from build123d import *

# Parameters (mm, degrees)
FILLET1_R = 1.524
FILLET2_R = 0.508


with BuildPart() as part:
    # Sketch3 → Revolve1 (revolve)
    with BuildSketch(Plane(origin=(0, 0, 0), x_dir=(0, 0, -1), z_dir=(1, 0, 0))):
        Polygon((-35.9918, -34.3535), (35.9918, -34.3535), (35.9918, -30.3149), (1.1938, -30.3149), (1.1938, -29.1973), (-1.1938, -29.1973), (-1.1938, -30.3149), (-35.9918, -30.3149), align=None)
    revolve(axis=Axis((0, 0, 35.9918), (0, 0, -1)))

    # Fillet1
    fillet1_edges = [part.edges().sort_by_distance(p)[0] for p in [
        (0, 30.3149, -35.9918),
        (0, 30.3149, 35.9918),
    ]]
    fillet(fillet1_edges, radius=FILLET1_R)

    # Fillet2
    fillet2_edges = [part.edges().sort_by_distance(p)[0] for p in [
        (0, 30.3149, -1.1938),
        (0, 30.3149, 1.1938),
    ]]
    fillet(fillet2_edges, radius=FILLET2_R)


solid = part.part
Could you check a few things on this model? Use its own coordinates, in mm. A direction names the side the tool comes from. Give positions to 0.01 mm unless a question says otherwise; leave off trailing zeros. Loops run counter-clockwise (first coordinate to the right, second up) from the corner with the lowest first, then second, coordinate; pieces in that order, holes last. Notation, with made-up numbers: (-29.75, 13) -> (16.25, 13) arc R33 cw to (16.25, 50) -> close; hole circle Ø9 at (71.25, 32). An arc over 180 degrees is marked (long way). Answer as CSV lines item,"result". Start each with the question number.
(1) If we section it at C-C on z = 10.5: Write out the boundary of the cut face in (x, y).
(2) Which directions (+Z, -Z, +X, -X, +Y, -Y) give clear straight access to the entire face, cutting with the end or side of a thin tool? Please do faces 1 (the flat face through (21.9, -19.7, -1.194)), 2 (the cylindrical face through (-28.95, 3.8, 0.02)), 3 (the cylindrical face through (29.594, 6.572, 18.314)).
(3) I need wall thicknesses on probe 1 along Y at (x, z) = (0, 19); probe 2 along Y at (x, z) = (0, 0). Which ranges of each line are inside material? Lowest first, please.
(4) We'd pull the mould along X, two halves only. Please class faces 4 (the cylindrical face through (33.537, 7.447, -0.504)), 5 (the flat face through (10, -30.4, -35.992)), 6 (the cylindrical face through (29.594, 6.572, -17.855)), 7 (the flat face through (21.9, 19.7, 1.194)): released by +X, released by -X, zero draft, split by the parting line, or undercut.
(5) If we section it at A-A on y = 0: Write out the boundary of the cut face in (x, z).
(6) I'm going to push flat-ended pins straight in: pin 1 Ø4 at (x, z) = (-14, -10) entering from +Y; pin 2 Ø2 at (y, z) = (7, -22.5) entering from -X; pin 3 Ø1 at (x, y) = (23, -15) entering from -Z; pin 4 Ø1 at (y, z) = (22.5, -17) entering from -X. Where does each tip first touch, or does it pass through?
Computed:
1,outline,"circle Ø68.71 at (0, 0); hole circle Ø60.63 at (0, 0)"
2,face 1,"-Z"
2,face 2,"+Z, -Z"
2,face 3,"+Z"
3,probe 1,"y = -34.35 to -30.31, 30.31 to 34.35"
3,probe 2,"y = -34.35 to -29.2, 29.2 to 34.35"
4,face 4,"split by the parting line"
4,face 5,"zero draft"
4,face 6,"undercut"
4,face 7,"undercut"
5,outline,"(-34.35, -35.99) -> (-31.84, -35.99) arc R1.52 ccw to (-30.31, -34.47) -> (-30.31, -1.7) arc R0.51 cw to (-29.81, -1.19) -> (-29.2, -1.19) -> (-29.2, 1.19) -> (-29.81, 1.19) arc R0.51 cw to (-30.31, 1.7) -> (-30.31, 34.47) arc R1.52 ccw to (-31.84, 35.99) -> (-34.35, 35.99) -> close; (29.2, -1.19) -> (29.81, -1.19) arc R0.51 cw to (30.31, -1.7) -> (30.31, -34.47) arc R1.52 ccw to (31.84, -35.99) -> (34.35, -35.99) -> (34.35, 35.99) -> (31.84, 35.99) arc R1.52 ccw to (30.31, 34.47) -> (30.31, 1.7) arc R0.51 cw to (29.81, 1.19) -> (29.2, 1.19) -> close"
6,pin 1,"stops at y = 32.19"
6,pin 2,"stops at x = -33.83"
6,pin 3,"passes through"
6,pin 4,"stops at x = -26.38"
